from build123d import *

# Parameters (mm, degrees)
F1_DEPTH = 90
F2_DEPTH = 5


with BuildPart() as f1:
    # F0 (on Front) → F1 (new body)
    with BuildSketch(Plane.XZ):
        Polygon((-27, 12), (-32, 12), (-32, 0), (0, 0), (32, 0), (32, 12), (27, 12), (27, 5), (0, 5), (-27, 5), align=None)
    extrude(amount=F1_DEPTH)

    # F0 (on Front) → F2 (join)
    with BuildSketch(Plane.XZ):
        Polygon((-27, 12), (-32, 12), (-32, 0), (0, 0), (32, 0), (32, 12), (27, 12), (27, 5), (0, 5), (-27, 5), align=None)
        Polygon((27, 12), (-27, 12), (-27, 5), (0, 5), (27, 5), align=None)
    extrude(amount=-F2_DEPTH)


solid = f1.part
Can you work these out from the model? Positions are in its coordinate system, mm. A direction names the side the tool comes from. Coordinates: 2 decimals unless noted, no trailing zeros. Order: outer loops, then holes, each group sorted by start corner. A loop starts at its lowest first (then second) coordinate and runs counter-clockwise, first axis right, second up. Notation, with made-up numbers: (41, 28) -> (98, 28) arc R9 cw to (98, 32) -> close; hole circle Ø7 at (14.5, 65). An arc over 180 degrees is marked (long way). Use one line per item in the form item = value.
Q1. We'd pull the mould along X, two halves only. Please class faces 1 (the face through (-32, -43, 6)), 2 (the face through (0, 0, 9)), 3 (the face through (0, -90, 3)): released by +X, released by -X, zero draft, split by the parting line, or undercut.
From the geometry:
face_1 = released by -X
face_2 = undercut
face_3 = zero draft
Q2. Imagine slicing it at A-A, the plane z = 9. List the corners of the cut face in (x, y) for me, then the cut area to 3 significant figures.
From the geometry:
outline = (-32, -90) -> (-27, -90) -> (-27, 0) -> (27, 0) -> (27, -90) -> (32, -90) -> (32, 5) -> (-32, 5) -> close
area = 1,220 mm²
Q3. Imagine slicing it at C-C, the plane x = -3. List the corners of the cut face in (y, z) for me.
From the geometry:
outline = (-90, 0) -> (5, 0) -> (5, 12) -> (0, 12) -> (0, 5) -> (-90, 5) -> close
Q4. Will this pin go through, and if not, where does the flat tip stop? P1, Ø3, axis at x = -22.5, y = -30.5, coming from the +Z side.
From the geometry:
P1 = 5
Q5. Imagine slicing it at B-B, the plane y = -3.5. List the corners of the cut face in (x, z) for me, then the cut area to 3 significant figures.
From the geometry:
outline = (-32, 0) -> (32, 0) -> (32, 12) -> (27, 12) -> (27, 5) -> (-27, 5) -> (-27, 12) -> (-32, 12) -> close
area = 390 mm²
Q6. I need wall thicknesses on L1, parallel to X at y = -70, z = 10.5; L2, parallel to Z at x = 14, y = -39. Which ranges of each line are inside material? Lowest first, please.
From the geometry:
L1 = -32 to -27, 27 to 32
L2 = 0 to 5
Q7. Which directions (+Z, -Z, +X, -X, +Y, -Y) give clear straight access to the entire face, cutting with the end or side of a thin tool? Please do faces 4 (the face through (0, -44, 5)), 5 (the face through (0, -43, 0)).
From the geometry:
face_4 = +Z, -Y
face_5 = -Z, +X, -X, +Y, -Y
